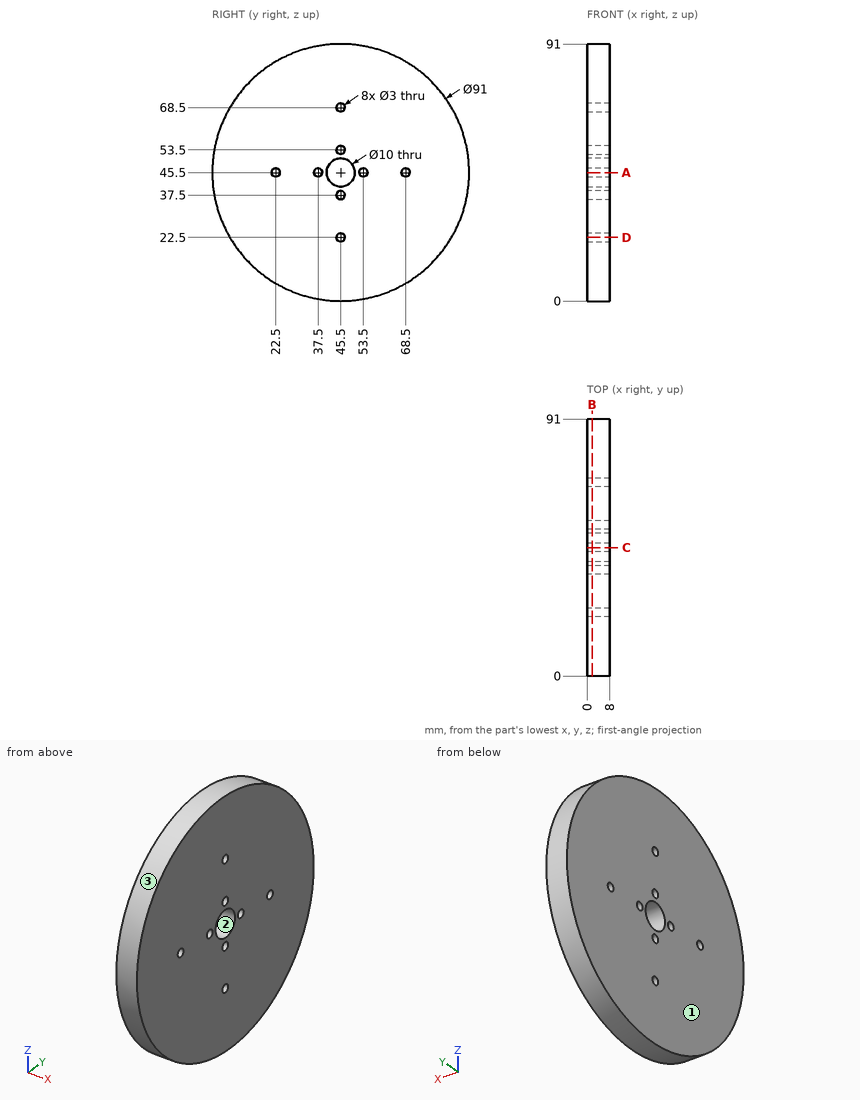
Design review of the part shown in the three views and the two pictorial views. Dimensions are in mm from the part's minimum x, y and z. Give positions to 0.01 mm unless a question says otherwise; leave off trailing zeros. Write each loop counter-clockwise with the first axis right and the second up, starting at its lowest first coordinate (ties: lowest second). Pieces come first, ordered by that corner, then holes.
Item 1: Take a section at D-D (z = 22.5). Give the boundary of the cut face in (x, y).
Item 2: The part is to be moulded in two halves that separate along Z. For the marked faces 1, 2 and 3, say which applies: +Z half, -Z half, draft (parallel to the pull), parting line (faces both ways), or undercut.
Item 3: Wall thickness on probe 1 along Y at (x, z) = (4.25, 45.5); probe 2 along Z at (x, y) = (2, 44.5); probe 3 along Y at (x, z) = (3, 37.5): over which ranges is each line inside the solid? List them lowest first.
Item 4: Take a section at A-A (z = 45.5). Give the boundary of the cut face in (x, y).
Item 5: Insertion check: P1, Ø1, axis at x = 1, y = 69.5, coming from the -Z side; P2, Ø2.5, axis at y = 45.5, z = 53.5, coming from the -X side; P3, Ø1, axis at x = 4, z = 22.5, coming from the -Y side; P4, Ø1.5, axis at x = 2.5, y = 21.5, coming from the +Z side. Each pin has a flat end and moves straight along its axis. Give the tip position at first contact, or say it passes through.
Item 6: Take a section at B-B (x = 1.75). Give the number of separate pieces and of enclosed holes in the cut face, and give its area (3 significant figures).
Established:
1. outline: (0, 6.24) - (8, 6.24) - (8, 44) - (0, 44) - close; (0, 47) - (8, 47) - (8, 84.76) - (0, 84.76) - close
2. face 1: draft
2. face 2: undercut
2. face 3: parting line
3. probe 1: y = 0 to 21, 24 to 36, 39 to 40.5, 50.5 to 52, 55 to 67, 70 to 91
3. probe 2: z = 0.01 to 21.38, 23.62 to 36.38, 38.62 to 40.6, 50.4 to 52.38, 54.62 to 67.38, 69.62 to 90.99
3. probe 3: y = 0.71 to 44, 47 to 90.29
4. outline: (0, 0) - (8, 0) - (8, 21) - (0, 21) - close; (0, 24) - (8, 24) - (8, 36) - (0, 36) - close; (0, 39) - (8, 39) - (8, 40.5) - (0, 40.5) - close; (0, 50.5) - (8, 50.5) - (8, 52) - (0, 52) - close; (0, 55) - (8, 55) - (8, 67) - (0, 67) - close; (0, 70) - (8, 70) - (8, 91) - (0, 91) - close
5. P1: stops at z = 6.54
5. P2: passes through
5. P3: stops at y = 5.95
5. P4: stops at z = 84.61
6. separate pieces: 1
6. enclosed holes: 9
6. area: 6,370 mm2
